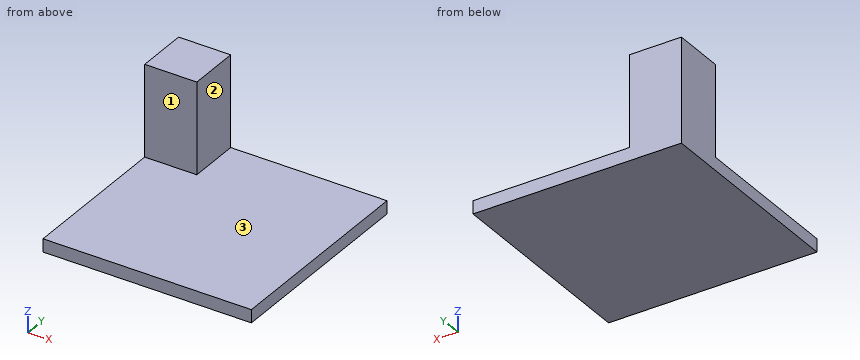
```python
from build123d import *

# Parameters (mm, degrees)
F1_DEPTH = 1.5875
F0_W     = 6.35
F0_H     = 6.35
F2_DEPTH = 12.7


# Not quite as in the source:
# - a length typed as a fraction of an inch, garbled in the dataset ("3 / 203.2 mm" for 3/8 in), is restored


with BuildPart() as f1:
    # F0 (on Top) → F1 (new body)
    with BuildSketch(Plane.XY):
        Polygon((-12.7, -12.7), (12.7, -12.7), (12.7, 12.7), (-6.35, 12.7), (-6.35, 6.35), (-12.7, 6.35), align=None)
    extrude(amount=F1_DEPTH)

    # F0 (on Top) → F2 (join)
    with BuildSketch(Plane.XY):
        with Locations((-9.525, 9.525)):
            Rectangle(F0_W, F0_H)
    extrude(amount=F2_DEPTH)


solid = f1.part
```
Could you check a few things on this model? Use its own coordinates, in mm. Face numbers are marked on the shaded views. A direction names the side the tool comes from. Give positions to 0.01 mm unless a question says otherwise; leave off trailing zeros. Order: outer loops, then holes, each group sorted by start corner. A loop starts at its lowest first (then second) coordinate and runs counter-clockwise, first axis right, second up.
Q1. Suppose I cut it at C-C, the plane z = 6. Write out the boundary of the cut face in (x, y), and give its area (3 significant figures).
Q2. For the marked faces 1, 2 and 3, which set-ups out of +Z, -Z, +X, -X, +Y, -Y let a thin tool reach every point of the face, with its end or its side?
Q3. I'm going to push flat-ended pins straight in: P1, Ø7, axis at y = 9, z = 5.5, coming from the +X side; P2, Ø7, axis at x = -11, z = 8.5, coming from the -Y side. Where does each tip first touch, or does it pass through?
Q4. Suppose I cut it at D-D, the plane y = 4. Write out the boundary of the cut face in (x, z).
Q5. If I drill on line 1 along Z through (x, y) = (8.75, -3); line 2 along X through (y, z) = (11.25, 2), over which ranges is the centre line in solid material (lowest first)?
Q6. Suppose I cut it at B-B, the plane y = 8.25. Write out the boundary of the cut face in (x, z).
Q7. Suppose I cut it at A-A, the plane x = -8. Write out the boundary of the cut face in (y, z), and give its area (3 significant figures).
Solution:
1. outline: (-12.7, 6.35) - (-6.35, 6.35) - (-6.35, 12.7) - (-12.7, 12.7) - close
1. area: 40.3 mm2
2. face 1: +Z, +X, -X, -Y
2. face 2: +Z, +X, +Y, -Y
2. face 3: +Z, +X, -Y
3. P1: stops at x = -6.35
3. P2: stops at y = 6.35
4. outline: (-12.7, 0) - (12.7, 0) - (12.7, 1.59) - (-12.7, 1.59) - close
5. line 1: z = 0 to 1.59
5. line 2: x = -12.7 to -6.35
6. outline: (-12.7, 0) - (12.7, 0) - (12.7, 1.59) - (-6.35, 1.59) - (-6.35, 12.7) - (-12.7, 12.7) - close
7. outline: (-12.7, 0) - (12.7, 0) - (12.7, 12.7) - (6.35, 12.7) - (6.35, 1.59) - (-12.7, 1.59) - close
7. area: 111 mm2
